Read the model definition and answer for the solid it produces. Units are mm, in the model's axes. Face numbers are marked on the shaded views. A direction names the side the tool comes from. Coordinates: 2 decimals unless noted, no trailing zeros. Write each loop counter-clockwise with the first axis right and the second up, starting at its lowest first coordinate (ties: lowest second). Pieces come first, ordered by that corner, then holes.
Item 1: Each of these flat-tipped pins is pushed along its axis until it touches: P1, Ø1.3, axis at x = 10.5, y = 5, coming from the -Z side; P2, Ø3, axis at x = -17.5, y = 10, coming from the -Z side; P3, Ø1.2, axis at y = 3.5, z = 7.5, coming from the -X side; P4, Ø8.5, axis at x = 14.5, y = -20.8, coming from the +Z side. Where does it stop, or does it pass through?
Item 2: Section C-C (x = 14.5) is taken. Give the vertices of the cut face in (y, z).
Item 3: Section A-A (z = 2.25) is taken. State how many separate pieces and enclosed holes the cut face has, then the cut area to 3 significant figures.
Item 4: Straight lines are drawn through the part: probe 1 along Y at (x, z) = (14.5, 1.95); probe 2 along Y at (x, z) = (-14.5, 2.65); probe 3 along Y at (x, z) = (-17.5, 6.25). For each, find the intervals that lie inside material, in ascending order.
Item 5: A tool of negligible diameter and unlimited length cuts with its end or side. For the marked faces 5, 6, 7, 8 and 9, from which of +Z, -Z, +X, -X, +Y, -Y can it reach the whole face along a straight path? Write none if from no direction.
Item 6: Section D-D (x = -4) is taken. Give the vertices of the cut face in (y, z).
Item 7: Determine the mould class of the marked faces 1, 2, 3 and 4 for opening direction X: released by +X, released by -X, zero draft, split by the parting line, or undercut.
Item 8: Section B-B (y = 10) is taken. Give the vertices of the cut face in (x, z), then the cut area to 3 significant figures.
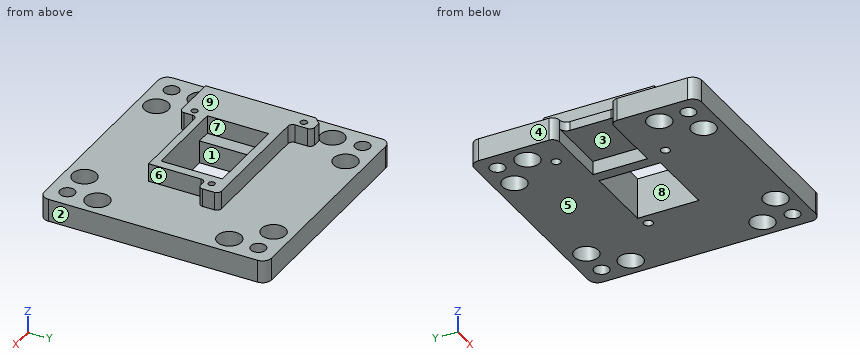
Autodesk Inventor part; units mm, degrees
ref_plane "Work Plane1" through (-29.7499, -21.1921, 9) normal (0, 0, -1) x (-0.4175, 0.9087, 0)
ref_plane "YZ Plane" through (0, 0, 0) normal (1, 0, 0) x (0, 1, 0)
ref_plane "XZ Plane" through (0, 0, 0) normal (0, 1, 0) x (-1, 0, 0)
sketch "Sketch1" plane through (0, 0, 0) normal (0, 0, 1) x (1, 0, 0)
  line L0 (-25, 25) -> (25, 25)
  line L1 (25, 25) -> (25, -25)
  line L2 (25, -25) -> (-25, -25)
  line L3 (-25, -25) -> (-25, 25)
  line L4 (-25, 25) -> (25, -25) construction
  line L5 (25, 25) -> (-25, -25) construction
  circle A0 centre (0, 0) radius 2.5
  circle A1 centre (-20.8, -14.5) radius 2.65
  circle A2 centre (-14.5, -20.8) radius 2.65
  circle A3 centre (-20.8, 14.5) radius 2.65
  circle A4 centre (20.8, -14.5) radius 2.65
  circle A5 centre (20.8, 14.5) radius 2.65
  circle A6 centre (-14.5, 20.8) radius 2.65
  circle A7 centre (14.5, -20.8) radius 2.65
  circle A8 centre (14.5, 20.8) radius 2.65
  dimension "d0" = 50
  dimension "d1" = 50
  dimension "d2" = 5
  dimension "d5" = 5.3
  dimension "d6" = 4.2
  dimension "d8" = 10.5
  dimension "d11" = 29
  dimension "d14" = 41.6
extrude "Extrusion1" add sketch "Sketch1" along normal blind 5
fillet "Fillet1" radius 2 4 edges at (-25, 25, 2.5) (25, 25, 2.5) (-25, -25, 2.5) (25, -25, 2.5)
sketch "Sketch2" plane through (0, 0, 5) normal (0, 0, 1) x (1, 0, 0)
  arc A0 (23, -25) -> (25, -23) centre (23, -23) ccw
  line L0 (25, -23) -> (25, 23)
  arc A1 (25, 23) -> (23, 25) centre (23, 23) ccw
  line L1 (23, 25) -> (-23, 25)
  arc A2 (-23, 25) -> (-25, 23) centre (-23, 23) ccw
  line L2 (-25, 23) -> (-25, -23)
  arc A3 (-25, -23) -> (-23, -25) centre (-23, -23) ccw
  line L3 (-23, -25) -> (23, -25)
  circle A4 centre (14.5, 20.8) radius 2.65
  circle A5 centre (-14.5, 20.8) radius 2.65
  circle A6 centre (14.5, -20.8) radius 2.65
  circle A7 centre (20.8, 14.5) radius 2.65
  circle A8 centre (20.8, -14.5) radius 2.65
  circle A9 centre (-20.8, 14.5) radius 2.65
  circle A10 centre (-14.5, -20.8) radius 2.65
  circle A11 centre (-20.8, -14.5) radius 2.65
  circle A12 centre (0, 0) radius 2.5
  line L4 (21, -21) -> (-21, -21)
  line L5 (-21, -21) -> (-21, 21)
  line L6 (-21, 21) -> (21, 21)
  line L7 (21, 21) -> (21, -21)
  line L8 (21, -21) -> (-21, 21) construction
  line L9 (-21, -21) -> (21, 21) construction
  circle A13 centre (-28.6, 21.06) radius 1.55
  dimension "d18" = 42
  dimension "d19" = 42
hole "Hole1" at (-21, 21, 5) at (21, 21, 5) at (21, -21, 5) at (-21, -21, 5) direction (0, 0, -1) diameter 3.3 end through all both
sketch "Sketch4" plane through (0, 0, 0) normal (0, 0, -1) x (-1, 0, 0)
  line L0 (15, 15) -> (15, -15) construction
  line L1 (-15, 15) -> (15, 15) construction
  line L2 (15, -15) -> (-15, -15) construction
  line L3 (-15, -15) -> (-15, 15) construction
  circle A0 centre (-21, -21) radius 1.65 construction
  circle A1 centre (21, 21) radius 1.65 construction
  circle A2 centre (-21, 21) radius 1.65 construction
  circle A3 centre (21, -21) radius 1.65 construction
  circle A4 centre (-14.5, 20.8) radius 2.65 construction
  circle A5 centre (14.5, 20.8) radius 2.65 construction
  circle A6 centre (-14.5, -20.8) radius 2.65 construction
  circle A7 centre (-20.8, 14.5) radius 2.65 construction
  circle A8 centre (-20.8, -14.5) radius 2.65 construction
  circle A9 centre (20.8, 14.5) radius 2.65 construction
  circle A10 centre (14.5, -20.8) radius 2.65 construction
  circle A11 centre (20.8, -14.5) radius 2.65 construction
  circle A12 centre (0, 0) radius 2.5 construction
  arc A13 (-25, -23) -> (-23, -25) centre (-23, -23) ccw construction
  line L4 (-23, -25) -> (23, -25) construction
  arc A14 (23, -25) -> (25, -23) centre (23, -23) ccw construction
  line L5 (25, -23) -> (25, 23) construction
  arc A15 (25, 23) -> (23, 25) centre (23, 23) ccw construction
  line L6 (23, 25) -> (-23, 25) construction
  arc A16 (-23, 25) -> (-25, 23) centre (-23, 23) ccw construction
  line L7 (-25, 23) -> (-25, -23) construction
  line L8 (-25, -23) -> (-25, 23) construction
  line L9 (-25, 0) -> (25, 0) construction
  line L10 (25, 23) -> (25, -23) construction
  line L11 (10, 6) -> (15, 6) construction
  line L12 (15, 6) -> (15, -6) construction
  line L13 (15, -6) -> (10, -6) construction
  line L14 (10, -6) -> (10, 6) construction
  line L15 (10, 6) -> (25, 6)
  line L16 (25, 6) -> (25, -6)
  line L17 (25, -6) -> (10, -6)
  line L18 (10, -6) -> (10, 6)
  dimension "d34" = 5
  dimension "d35" = 12
extrude "Extrusion2" cut sketch "Sketch4" against normal blind 3
sketch "Sketch5" plane through (0, 0, 3) normal (0, 0, -1) x (-1, 0, 0)
  line L0 (10, 6) -> (25, 6)
  line L1 (10, -6) -> (10, 6)
  line L2 (25, -6) -> (10, -6)
  line L3 (25, 6) -> (25, -6)
  line L4 (25, 6) -> (25, -6)
  line L5 (25, -6) -> (10, -6)
  line L6 (25, 6) -> (22, 6)
  line L7 (22, 6) -> (22, -6)
  line L8 (22, -6) -> (25, -6)
  line L9 (25, -6) -> (25, 6)
  point P0 (0, 0)
  dimension "d38" = 3
extrude "Extrusion3" cut sketch "Sketch5" against normal up to surface (2 mm away) contours L0 L3 L2 L7
fillet "Fillet2" radius 1.5 4 edges at (-25, 6, 2.5) (-25, -6, 2.5) (-22, 6, 4) (-22, -6, 4)
sketch "Sketch6" plane through (0, 0, 5) normal (0, 0, 1) x (1, 0, 0)
  arc A0 (-15.8555, 11.7) -> (-16.8555, 12.7) centre (-16.8555, 11.7) ccw
  line L0 (-16.8555, 12.7) -> (-20, 12.7)
  line L1 (-20, 12.7) -> (-20, -13)
  line L2 (-20, -13) -> (-10.4723, -13)
  arc A1 (-10.4723, -13) -> (-9.4723, -12) centre (-10.4723, -12) ccw
  line L3 (-9.4723, -12) -> (-9.4723, -10.1376)
  arc A2 (-8.4723, -9.1376) -> (-9.4723, -10.1376) centre (-8.4723, -10.1376) ccw
  line L4 (-8.4723, -9.1376) -> (10, -9.1376)
  line L5 (10, -9.1376) -> (10, 2.397)
  arc A3 (11, 3.397) -> (10, 2.397) centre (11, 2.397) ccw
  line L6 (11, 3.397) -> (12, 3.397)
  arc A4 (12, 3.397) -> (13, 4.397) centre (12, 4.397) ccw
  line L7 (13, 4.397) -> (13, 6.9624)
  arc A5 (13, 6.9624) -> (12, 7.9624) centre (12, 6.9624) ccw
  line L8 (12, 7.9624) -> (-14.8555, 7.9624)
  arc A6 (-15.8555, 8.9624) -> (-14.8555, 7.9624) centre (-14.8555, 8.9624) ccw
  line L9 (-15.8555, 8.9624) -> (-15.8555, 11.7)
  line L10 (-7.5, 6) -> (8, 6)
  line L11 (8, 6) -> (8, -7.5)
  line L12 (8, -7.5) -> (-7.5, -7.5)
  line L13 (-7.5, -7.5) -> (-7.5, 6)
  circle A7 centre (-17.5, 10) radius 1 construction
  circle A8 centre (-11, -10.5) radius 1 construction
  circle A9 centre (10.5, 5) radius 1 construction
  line L14 (-18.5716, 12.7) -> (-20, 11.2716)
  line L15 (-18.5716, 12.7) -> (-16.5515, 12.7) construction
  line L16 (8, 6) -> (-10.6432, 6)
  line L17 (-10.6432, 6) -> (-10.6432, -7.5)
  line L18 (-10.6432, -7.5) -> (8, -7.5)
  line L19 (8, -7.5) -> (8, 6)
  circle A10 centre (-17.5, 10) radius 0.75
  circle A11 centre (10.5, 5) radius 0.7
  circle A12 centre (-11, -10.5) radius 0.7
  point P0 (0, 0)
  dimension "d42" = 135
  dimension "d47" = 1.5
  dimension "d48" = 1.4
  dimension "d49" = 1.4
ref_plane "Work Plane1" through (-29.7499, -21.1921, 9) normal (0, 0, -1) x (-0.4175, 0.9087, 0)
extrude "Extrusion4" add sketch "Sketch6" along normal up to surface (4 mm away) contours L9 A6 L8 A5 L7 A4 L6 A3 L5 L4 A2 L3 A1 L2 L1 L14 L0 A0
sketch "Sketch7" plane through (0, 0, 5) normal (0, 0, 1) x (1, 0, 0)
  point P0 (0, 0)
sketch "Sketch8" plane through (0, 0, 5) normal (0, 0, 1) x (1, 0, 0)
  arc A0 (-15.8555, 11.7) -> (-16.8555, 12.7) centre (-16.8555, 11.7) ccw
  line L0 (-16.8555, 12.7) -> (-20, 12.7)
  line L1 (-20, 12.7) -> (-20, -13)
  line L2 (-20, -13) -> (-10.4723, -13)
  arc A1 (-10.4723, -13) -> (-9.4723, -12) centre (-10.4723, -12) ccw
  line L3 (-9.4723, -12) -> (-9.4723, -10.1376)
  arc A2 (-8.4723, -9.1376) -> (-9.4723, -10.1376) centre (-8.4723, -10.1376) ccw
  line L4 (-8.4723, -9.1376) -> (10, -9.1376)
  line L5 (10, -9.1376) -> (10, 2.397)
  arc A3 (11, 3.397) -> (10, 2.397) centre (11, 2.397) ccw
  line L6 (11, 3.397) -> (12, 3.397)
  arc A4 (12, 3.397) -> (13, 4.397) centre (12, 4.397) ccw
  line L7 (13, 4.397) -> (13, 6.9624)
  arc A5 (13, 6.9624) -> (12, 7.9624) centre (12, 6.9624) ccw
  line L8 (12, 7.9624) -> (-14.8555, 7.9624)
  arc A6 (-15.8555, 8.9624) -> (-14.8555, 7.9624) centre (-14.8555, 8.9624) ccw
  line L9 (-15.8555, 8.9624) -> (-15.8555, 11.7)
  line L10 (-7.5, 6) -> (8, 6)
  line L11 (8, 6) -> (8, -7.5)
  line L12 (8, -7.5) -> (-7.5, -7.5)
  line L13 (-7.5, -7.5) -> (-7.5, 6)
  circle A7 centre (-17.5, 10) radius 1
  circle A8 centre (-11, -10.5) radius 1
  circle A9 centre (10.5, 5) radius 1
  point P0 (0, 0)
extrude "Extrusion5" cut sketch "Sketch8" against normal blind 10 contours L10 L11 L12 L13 | A7 | A8 | A9
properties part number "30_IM_TopPlate_KES400A_holder_v3"
Established:
1. P1: passes through
1. P2: stops at z = 0
1. P3: stops at x = -20
1. P4: stops at z = 5
2. outline: (-25, 0) - (-23.45, 0) - (-23.45, 5) - (-25, 5) - close; (-18.15, 0) - (18.15, 0) - (18.15, 5) - (-18.15, 5) - close; (23.45, 0) - (25, 0) - (25, 5) - (23.45, 5) - close
3. separate pieces: 1
3. enclosed holes: 16
3. area: 1,890 mm2
4. probe 1: y = -25 to -23.45, -18.15 to 18.15, 23.45 to 25
4. probe 2: y = -25 to -23.45, -18.15 to -6, 6 to 18.15, 23.45 to 25
4. probe 3: y = -13 to 9.25, 10.75 to 12.7
5. face 5: -Z, +X, -X, +Y, -Y
5. face 6: +Z, +X, -Y
5. face 7: +Z
5. face 8: +Z, -Z
5. face 9: +Z, +X, -X, +Y, -Y
6. outline: (-25, 0) - (-7.5, 0) - (-7.5, 9) - (-9.14, 9) - (-9.14, 5) - (-25, 5) - close; (6, 0) - (25, 0) - (25, 5) - (7.96, 5) - (7.96, 9) - (6, 9) - close
7. face 1: undercut
7. face 2: released by +X
7. face 3: zero draft
7. face 4: released by -X
8. outline: (-25, 0) - (-18.5, 0) - (-18.5, 5) - (-18.25, 5) - (-18.25, 9) - (-20, 9) - (-20, 5) - (-25, 5) - close; (-16.75, 5) - (-16.5, 5) - (-16.5, 0) - (25, 0) - (25, 5) - (-15.86, 5) - (-15.86, 9) - (-16.75, 9) - close
8. area: 251 mm2
